Input: part model. Units: mm. Frame: model coordinates. A direction names the side the tool comes from. Give positions to 0.01 mm unless a question says otherwise; leave off trailing zeros. Loops run counter-clockwise (first coordinate to the right, second up) from the corner with the lowest first, then second, coordinate; pieces in that order, holes last. Notation, with made-up numbers: (14, 89) - (47, 89) arc R24 cw to (47, 100) - close; hole circle Ø10 at (-26, 9). An arc over 180 degrees is marked (long way). Answer as a JSON object with one key per item and string values. Group by question number.
(1) Section query A-A (x = 0). Return loops of the section in (y, z).
(2) Material intervals for L1, parallel to X at y = 79.5, z = 3.75; L2, parallel to Y at x = 90, z = 7; L3, parallel to Y at x = -143.1, z = 8.25, sorted ascending.
(3) Mould query, pull axis Y, two halves, no side actions, for faces 1 (the flat face through (-150.6, 0, 6)), 2 (the cylindrical face through (-22.025, -99.184, 6.261)), 3 (the cylindrical face through (-116.823, -18.743, 6.439)). Classes: +Y half, -Y half, draft (parallel to the pull), parting line (faces both ways), or undercut.
(4) Section query B-B (y = 39). Return loops of the section in (x, z), plus the area to 3 significant figures.
(5) Section query C-C (z = 6.5). Count the separate pieces of the cut face and the enclosed holes in it, plus the area to 3 significant figures.
(6) Access query for faces 4 (the flat face through (-133, 17, 6)), 5 (the flat face through (-132, -17, 6)), 6 (the flat face through (133, -17, 6)). Directions: +Z, -Z, +X, -X, +Y, -Y. A direction counts if a zero-diameter tool reaches every point of the face in a straight line with its end or side. Return the directions, or none.
(7) Pin query (flat end, axial travel): P1, Ø6.5, axis at x = 131, z = 6.5, coming from the -Y side; P2, Ø2, axis at x = 80, z = 7, coming from the +Y side; P3, Ø1.5, axis at x = -89.5, z = 5.5, coming from the +Y side. Return the tip coordinate at first contact, or that it passes through.
```python
from build123d import *

# Parameters (mm, degrees)
SKETCH1_R           = 101.6
SKETCH1_R_2         = 2.1525
BOSS_EXTRUDE1_DEPTH = 12.7
FILLET1_R           = 7.5


with BuildPart() as part:
    # Sketch1 → Boss-Extrude1 (new body)
    with BuildSketch(Plane.XY):
        with BuildLine():
            Line((115.326459663, 17), (143.1, 17))
            ThreePointArc((143.1, 17), (148.403300859, 14.803300859), (150.6, 9.5))
            Line((150.6, 9.5), (150.6, -9.5))
            ThreePointArc((150.6, -9.5), (148.403300859, -14.803300859), (143.1, -17))
            Line((143.1, -17), (115.326459663, -17))
            ThreePointArc((115.326459663, -17), (0, -116.572691049), (-115.326459663, -17))
            Line((-115.326459663, -17), (-143.1, -17))
            ThreePointArc((-143.1, -17), (-148.403300859, -14.803300859), (-150.6, -9.5))
            Line((-150.6, -9.5), (-150.6, 9.5))
            ThreePointArc((-150.6, 9.5), (-148.403300859, 14.803300859), (-143.1, 17))
            Line((-143.1, 17), (-115.326459663, 17))
            ThreePointArc((-115.326459663, 17), (0, 116.572691049), (115.326459663, 17))
        make_face()
        Circle(SKETCH1_R, mode=Mode.SUBTRACT)
        with Locations((109.1, 0)):
            Circle(SKETCH1_R_2, mode=Mode.SUBTRACT)
        with Locations((106.71590324, -22.683165468)):
            Circle(SKETCH1_R_2, mode=Mode.SUBTRACT)
        with Locations((99.667809429, -44.37496776)):
            Circle(SKETCH1_R_2, mode=Mode.SUBTRACT)
        with Locations((88.263754086, -64.127371025)):
            Circle(SKETCH1_R_2, mode=Mode.SUBTRACT)
        with Locations((73.002149154, -81.07710046)):
            Circle(SKETCH1_R_2, mode=Mode.SUBTRACT)
        with Locations((54.55, -94.483371553)):
            Circle(SKETCH1_R_2, mode=Mode.SUBTRACT)
        with Locations((33.713754086, -103.760265928)):
            Circle(SKETCH1_R_2, mode=Mode.SUBTRACT)
        with Locations((11.404055343, -108.502338785)):
            Circle(SKETCH1_R_2, mode=Mode.SUBTRACT)
        with Locations((-11.404055343, -108.502338785)):
            Circle(SKETCH1_R_2, mode=Mode.SUBTRACT)
        with Locations((-33.713754086, -103.760265928)):
            Circle(SKETCH1_R_2, mode=Mode.SUBTRACT)
        with Locations((-54.55, -94.483371553)):
            Circle(SKETCH1_R_2, mode=Mode.SUBTRACT)
        with Locations((-73.002149154, -81.07710046)):
            Circle(SKETCH1_R_2, mode=Mode.SUBTRACT)
        with Locations((-88.263754086, -64.127371025)):
            Circle(SKETCH1_R_2, mode=Mode.SUBTRACT)
        with Locations((-99.667809429, -44.37496776)):
            Circle(SKETCH1_R_2, mode=Mode.SUBTRACT)
        with Locations((-106.71590324, -22.683165468)):
            Circle(SKETCH1_R_2, mode=Mode.SUBTRACT)
        with Locations((-109.1, 0)):
            Circle(SKETCH1_R_2, mode=Mode.SUBTRACT)
        with Locations((-106.71590324, 22.683165468)):
            Circle(SKETCH1_R_2, mode=Mode.SUBTRACT)
        with Locations((-99.667809429, 44.37496776)):
            Circle(SKETCH1_R_2, mode=Mode.SUBTRACT)
        with Locations((-88.263754086, 64.127371025)):
            Circle(SKETCH1_R_2, mode=Mode.SUBTRACT)
        with Locations((-73.002149154, 81.07710046)):
            Circle(SKETCH1_R_2, mode=Mode.SUBTRACT)
        with Locations((-54.55, 94.483371553)):
            Circle(SKETCH1_R_2, mode=Mode.SUBTRACT)
        with Locations((-33.713754086, 103.760265928)):
            Circle(SKETCH1_R_2, mode=Mode.SUBTRACT)
        with Locations((-11.404055343, 108.502338785)):
            Circle(SKETCH1_R_2, mode=Mode.SUBTRACT)
        with Locations((11.404055343, 108.502338785)):
            Circle(SKETCH1_R_2, mode=Mode.SUBTRACT)
        with Locations((33.713754086, 103.760265928)):
            Circle(SKETCH1_R_2, mode=Mode.SUBTRACT)
        with Locations((54.55, 94.483371553)):
            Circle(SKETCH1_R_2, mode=Mode.SUBTRACT)
        with Locations((73.002149154, 81.07710046)):
            Circle(SKETCH1_R_2, mode=Mode.SUBTRACT)
        with Locations((88.263754086, 64.127371025)):
            Circle(SKETCH1_R_2, mode=Mode.SUBTRACT)
        with Locations((99.667809429, 44.37496776)):
            Circle(SKETCH1_R_2, mode=Mode.SUBTRACT)
        with Locations((106.71590324, 22.683165468)):
            Circle(SKETCH1_R_2, mode=Mode.SUBTRACT)
        with Locations((133.6, 9.5)):
            Circle(SKETCH1_R_2, mode=Mode.SUBTRACT)
        with Locations((133.6, -9.5)):
            Circle(SKETCH1_R_2, mode=Mode.SUBTRACT)
        with Locations((143.1, 0)):
            Circle(SKETCH1_R_2, mode=Mode.SUBTRACT)
        with Locations((124.1, 0)):
            Circle(SKETCH1_R_2, mode=Mode.SUBTRACT)
        with Locations(Location((-143.1, 0, 0), (0, 0, 180))):
            Circle(SKETCH1_R_2, mode=Mode.SUBTRACT)
        with Locations(Location((-133.6, -9.5, 0), (0, 0, 180))):
            Circle(SKETCH1_R_2, mode=Mode.SUBTRACT)
        with Locations(Location((-124.1, 0, 0), (0, 0, 180))):
            Circle(SKETCH1_R_2, mode=Mode.SUBTRACT)
        with Locations(Location((-133.6, 9.5, 0), (0, 0, 180))):
            Circle(SKETCH1_R_2, mode=Mode.SUBTRACT)
    extrude(amount=BOSS_EXTRUDE1_DEPTH)

    # Fillet1
    fillet1_edges = [part.edges().sort_by_distance(p)[0] for p in [
        (115.326459663, 17, 6.35),
        (115.326459663, -17, 6.35),
        (-115.326459663, -17, 6.35),
        (-115.326459663, 17, 6.35),
    ]]
    fillet(fillet1_edges, radius=FILLET1_R)


solid = part.part
```
Recorded:
{
 "1": {"outline": "(-116.57, 0) - (-101.6, 0) - (-101.6, 12.7) - (-116.57, 12.7) - close; (101.6, 0) - (116.57, 0) - (116.57, 12.7) - (101.6, 12.7) - close"},
 "2": {"L1": "x = -85.26 to -74.47, -71.54 to -63.26, 63.26 to 71.54, 74.47 to 85.26", "L2": "y = -74.09 to -65.4, -62.86 to -47.14, 47.14 to 62.86, 65.4 to 74.09", "L3": "y = -17 to -2.15, 2.15 to 17"},
 "3": {"face 1": "draft", "face 2": "undercut", "face 3": "-Y half"},
 "4": {"outline": "(-109.86, 0) - (-93.82, 0) - (-93.82, 12.7) - (-109.86, 12.7) - close; (93.82, 0) - (109.86, 0) - (109.86, 12.7) - (93.82, 12.7) - close", "area": "407 mm^2"},
 "5": {"separate pieces": "1", "enclosed holes": "39", "area": "12,000 mm^2"},
 "6": {"face 4": "+Z, -Z, -X, +Y", "face 5": "+Z, -Z, -X, -Y", "face 6": "+Z, -Z, +X, -Y"},
 "7": {"P1": "stops at y = -17", "P2": "stops at y = 85.72", "P3": "stops at y = 75.58"}
}
